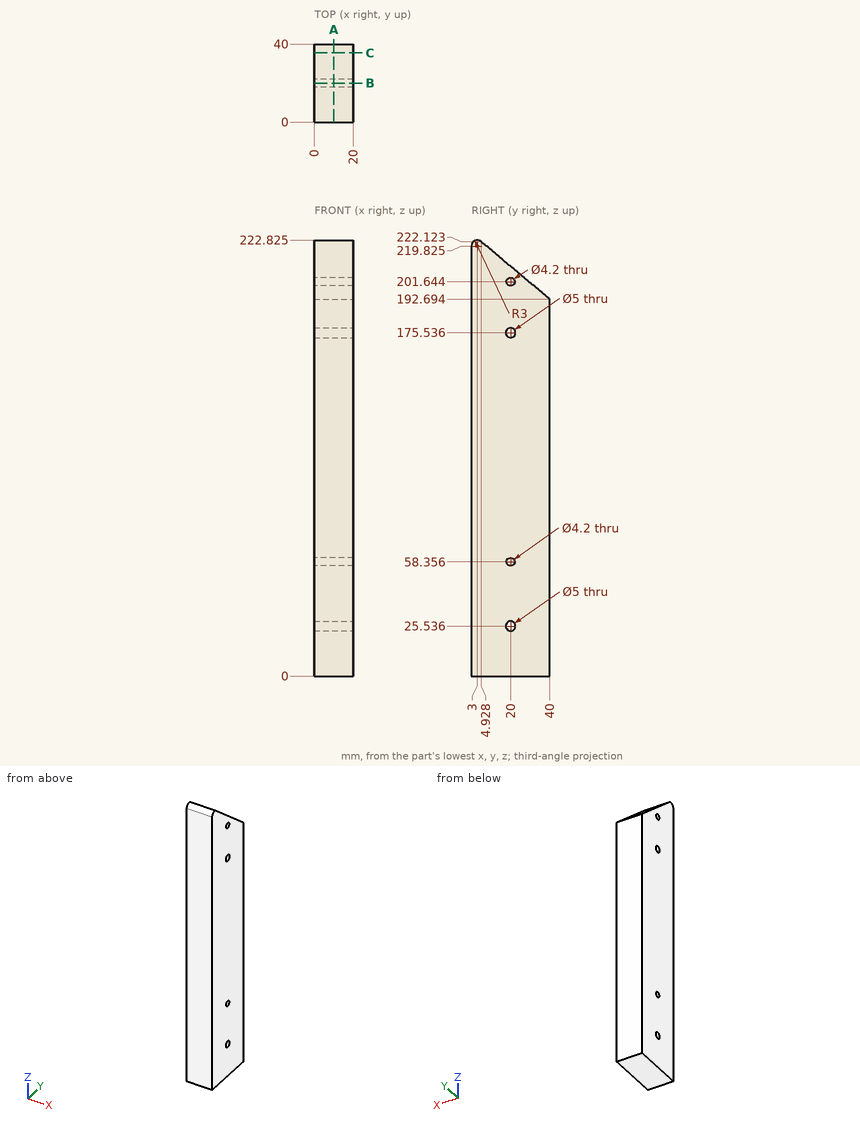
Design review of the part shown in the three views and the two pictorial views. Dimensions are in mm from the part's minimum x, y and z. Coordinates: 2 decimals unless noted, no trailing zeros. Write each loop counter-clockwise with the first axis right and the second up, starting at its lowest first coordinate (ties: lowest second). Pieces come first, ordered by that corner, then holes.
(1) Add section A-A on x = 10. Give the boundary of the cut face in (y, z) (1 decimal).
(2) Add section B-B on y = 20. Give the boundary of the cut face in (x, z) (1 decimal), then the cut area to 3 significant figures.
(3) Add section C-C on y = 35.5. Give the boundary of the cut face in (x, z).
(4) Wall thickness on probe 1 along Y at (x, z) = (14, 176); probe 2 along Y at (x, z) = (11, 58); probe 3 along Z at (x, y) = (17.75, 25.5): over which ranges is each line inside the solid? List them lowest first.
(5) For pin 1 Ø10 at (x, y) = (10.5, 28.5) entering from -Z; pin 2 Ø4.5 at (y, z) = (20, 25.54) entering from +X; pin 3 Ø8 at (x, y) = (5, 14) entering from +Z; pin 4 Ø3 at (x, y) = (4, 29.5) entering from +Z, all flat-tipped, find the tip position at first contact; note any pin that passes through.
Answer sheet:
1. outline: (0, 0) - (40, 0) - (40, 192.7) - (4.9, 222.1) arc R3 ccw to (0, 219.8) - close; hole circle Ø5 at (20, 25.5); hole circle Ø5 at (20, 175.5); hole circle Ø4.2 at (20, 58.4); hole circle Ø4.2 at (20, 201.6)
2. outline: (0, 0) - (20, 0) - (20, 23) - (0, 23) - close; (0, 28) - (20, 28) - (20, 56.3) - (0, 56.3) - close; (0, 60.5) - (20, 60.5) - (20, 173) - (0, 173) - close; (0, 178) - (20, 178) - (20, 199.5) - (0, 199.5) - close; (0, 203.7) - (20, 203.7) - (20, 209.5) - (0, 209.5) - close
2. area: 3,820 mm2
3. outline: (0, 0) - (20, 0) - (20, 196.47) - (0, 196.47) - close
4. probe 1: y = 0 to 17.54, 22.46 to 40
4. probe 2: y = 0 to 17.93, 22.07 to 40
4. probe 3: z = 0 to 204.86
5. pin 1: stops at z = 0
5. pin 2: passes through
5. pin 3: stops at z = 217.87
5. pin 4: stops at z = 202.76
